```python
from build123d import *

# Parameters (mm, degrees)
F0_W     = 82
F0_H     = 95
F1_DEPTH = 6
F3_DEPTH = 6.001
F4_R     = 12
F4_R_2   = 1.6
F4_R_3   = 2.1
F5_DEPTH = 6.001
F6_R     = 5


# Not quite as in the source:
# - a pattern or mirror of a feature is missing from the dataset's text; its kind, count and spacing are read off the source's solid


with BuildPart() as f1:
    # F0 (on Top) → F1 (new body)
    with BuildSketch(Plane.XY):
        Rectangle(F0_W, F0_H)
    extrude(amount=F1_DEPTH)

    # F2 (on face) → F3 (cut, through all)
    with BuildSketch(Plane.XY.offset(6)):
        Polygon((-41, -27.5), (-21, 24.5), (-21, 47.5), (-41, 47.5), align=None)
    f3 = extrude(amount=-F3_DEPTH, mode=Mode.SUBTRACT)

    # F3_copies: F3 across plane
    add(f3.mirror(Plane(origin=(0, 0, 0), x_dir=(0, 0, 1), z_dir=(1, 0, 0))), mode=Mode.SUBTRACT)

    # F4 (on face) → F5 (cut, through all)
    with BuildSketch(Plane.XY.offset(6)):
        with Locations((0, 26.5003114)):
            Circle(F4_R)
        with Locations((15.5, 42.0003114)):
            Circle(F4_R_2)
        with Locations((-15.5, 42.0003114)):
            Circle(F4_R_2)
        with Locations((15.5, 11.0003114)):
            Circle(F4_R_2)
        with Locations((-15.5, 11.0003114)):
            Circle(F4_R_2)
        with Locations((-30, -37.5003114)):
            Circle(F4_R_3)
        with Locations((0, -37.5003114)):
            Circle(F4_R_3)
        with Locations((30, -37.5003114)):
            Circle(F4_R_3)
    extrude(amount=-F5_DEPTH, mode=Mode.SUBTRACT)

    # F6
    f6_edges = [f1.edges().sort_by_distance(p)[0] for p in [
        (-41, -47.5, 3),
        (41, -47.5, 3),
        (-21, 47.5, 3),
        (21, 47.5, 3),
    ]]
    fillet(f6_edges, radius=F6_R)


solid = f1.part
```
Here's how the part is built. I have some questions about the finished solid (model axes, mm). A direction names the side the tool comes from. Round coordinates to 2 decimals unless told otherwise and drop trailing zeros. Order: outer loops, then holes, each group sorted by start corner. A loop starts at its lowest first (then second) coordinate and runs counter-clockwise, first axis right, second up. Notation, with made-up numbers: (79, 8.25) -> (117, 8.25) arc R21 cw to (117, 30.25) -> close; hole circle Ø9 at (17.25, 85.5). An arc over 180 degrees is marked (long way). Use a Markdown table: item, result. Add a question column.
(1) If we mould it in two halves opening along X, with no side actions, what happens to faces 1 (the face through (6.45, 36.62, 3.04)), 2 (the face through (-1, -10, 0)), 3 (the face through (41, -35, 3))? For each: released by +X, released by -X, zero draft, split by the parting line, or undercut.
(2) For faces 4 (the face through (-41, -35, 3)), 5 (the face through (21, 33, 3)), 6 (the face through (-21, 33, 3)), which set-ups out of +Z, -Z, +X, -X, +Y, -Y let a thin tool reach every point of the face, with its end or its side?
(3) Suppose I cut it at B-B, the plane x = 30. Please give me the cut outline in (y, z).
(4) For pin 1 Ø1.8 at (y, z) = (33, 4) entering from -X, with a flat end and sliding along its axis, tell me the tip position at first contact or that it passes through.
(5) Suppose I cut it at C-C, the plane y = 34. Please give me the cut outline in (x, z), and give its area (3 significant figures).
(6) I need wall thicknesses on line 1 along Y through (x, z) = (15.5, 1.75); line 2 along Y through (x, z) = (0, 2.8); line 3 along X through (y, z) = (41.5, 1.25). Which ranges of each line are inside material? Lowest first, please.
(7) Suppose I cut it at A-A, the plane x = 0. Please give me the cut outline in (y, z), and give its area (3 significant figures).
(8) Suppose I cut it at D-D, the plane z = 1.75. Count the separate pieces of the cut face and the enclosed holes in it, and give its area (3 significant figures).
Verdict:
| question | item | result |
|---|---|---|
| 1 | face 1 | undercut |
| 1 | face 2 | zero draft |
| 1 | face 3 | released by +X |
| 2 | face 4 | +Z, -Z, -X, +Y, -Y |
| 2 | face 5 | +Z, -Z, +X, +Y |
| 2 | face 6 | +Z, -Z, -X, +Y |
| 3 | outline | (-47.5, 0) -> (-39.6, 0) -> (-39.6, 6) -> (-47.5, 6) -> close; (-35.4, 0) -> (1.1, 0) -> (1.1, 6) -> (-35.4, 6) -> close |
| 4 | pin 1 | x = -21 |
| 5 | outline | (-21, 0) -> (-9.37, 0) -> (-9.37, 6) -> (-21, 6) -> close; (9.37, 0) -> (21, 0) -> (21, 6) -> (9.37, 6) -> close |
| 5 | area | 140 mm2 |
| 6 | line 1 | -47.5 to 9.4, 12.6 to 40.4, 43.6 to 47.5 |
| 6 | line 2 | -47.5 to -39.6, -35.4 to 14.5, 38.5 to 47.5 |
| 6 | line 3 | -21 to -17.02, -13.98 to 13.98, 17.02 to 21 |
| 7 | outline | (-47.5, 0) -> (-39.6, 0) -> (-39.6, 6) -> (-47.5, 6) -> close; (-35.4, 0) -> (14.5, 0) -> (14.5, 6) -> (-35.4, 6) -> close; (38.5, 0) -> (47.5, 0) -> (47.5, 6) -> (38.5, 6) -> close |
| 7 | area | 401 mm2 |
| 8 | separate pieces | 1 |
| 8 | enclosed holes | 8 |
| 8 | area | 5,280 mm2 |
